from build123d import *

# Parameters (mm, degrees)
SKETCH1_W           = 81
SKETCH1_H           = 75
SKETCH1_R           = 1.585
BOSS_EXTRUDE1_DEPTH = 6.35


with BuildPart() as part:
    # Sketch1 → Boss-Extrude1 (new body)
    with BuildSketch(Plane(origin=(0, 0, 0), x_dir=(1, 0, 0), z_dir=(0, 1, 0))):
        with Locations((40.5, 37.5)):
            Rectangle(SKETCH1_W, SKETCH1_H)
        with Locations(Location((13.5, 5, 0), (0, 0, 270))):  # turned: the seam where the file's is
            Circle(SKETCH1_R, mode=Mode.SUBTRACT)
        with BuildLine():
            Line((6.175, 40), (74.825, 40))
            ThreePointArc((74.825, 40), (77.07006403, 40.92993597), (78, 43.175))
            Line((78, 43.175), (78, 66.825))
            ThreePointArc((78, 66.825), (77.07006403, 69.07006403), (74.825, 70))
            Line((74.825, 70), (6.175, 70))
            ThreePointArc((6.175, 70), (3.92993597, 69.07006403), (3, 66.825))
            Line((3, 66.825), (3, 43.175))
            ThreePointArc((3, 43.175), (3.92993597, 40.92993597), (6.175, 40))
        make_face(mode=Mode.SUBTRACT)
        with BuildLine():
            Line((61.83, 6.585), (65.17, 6.585))
            ThreePointArc((65.17, 6.585), (66.755, 5), (65.17, 3.415))
            Line((65.17, 3.415), (61.83, 3.415))
            ThreePointArc((61.83, 3.415), (60.245, 5), (61.83, 6.585))
        make_face(mode=Mode.SUBTRACT)
    extrude(amount=BOSS_EXTRUDE1_DEPTH)


solid = part.part
The listing builds one solid part. Answer for the finished solid, in the listing's coordinates (mm). A direction names the side the tool comes from. Coordinates: 2 decimals unless noted, no trailing zeros. Write each loop counter-clockwise with the first axis right and the second up, starting at its lowest first coordinate (ties: lowest second). Pieces come first, ordered by that corner, then holes. Notation, with made-up numbers: (3, 87.25) - (8, 87.25) arc R36 ccw to (8, 125.25) - close; hole circle Ø2 at (88, 59.5). An arc over 180 degrees is marked (long way). Put each result on its own line as item: value.
1. A flat-ended cylindrical pin translates along its axis: pin 1 Ø1.9 at (x, z) = (13.5, -5) entering from +Y. Find the tip coordinate at first contact, or state that the pin passes through.
Answer sheet:
pin 1: passes through
2. A tool of negligible diameter and unlimited length cuts with its end or side. For faces 5 (the face through (40, 6.35, -30)), 6 (the face through (63, 3, -6.585)), from which of +Z, -Z, +X, -X, +Y, -Y can it reach the whole face along a straight path? Write none if from no direction.
Answer sheet:
face 5: +Z, -Z, +X, -X, +Y
face 6: +Y, -Y
3. The part is cut by section B-B on x = 13.5. Give the vertices of the cut face in (y, z) (3 decimals).
Answer sheet:
outline: (0, -75) - (6.35, -75) - (6.35, -70) - (0, -70) - close; (0, -40) - (6.35, -40) - (6.35, -6.585) - (0, -6.585) - close; (0, -3.415) - (6.35, -3.415) - (6.35, 0) - (0, 0) - close
4. Determine the mould class of faces 1 (the face through (81, 3, -37)), 2 (the face through (40, 3, 0)), 3 (the face through (64, 3, -3.415)), 4 (the face through (3.95, 3.13, -69.09)) for opening direction X: pulls with the +X half, pulls with the -X half, needs draft (parallel to the pull), parting line crosses it, or undercut.
Answer sheet:
face 1: pulls with the +X half
face 2: needs draft
face 3: undercut
face 4: undercut
5. The part is cut by section A-A on z = -5. Give the vertices of the cut face in (x, y) (3 decimals).
Answer sheet:
outline: (0, 0) - (11.915, 0) - (11.915, 6.35) - (0, 6.35) - close; (15.085, 0) - (60.245, 0) - (60.245, 6.35) - (15.085, 6.35) - close; (66.755, 0) - (81, 0) - (81, 6.35) - (66.755, 6.35) - close
6. The part is cut by section D-D on y = 3.25. Give the vertices of the cut face in (x, z) (3 decimals).
Answer sheet:
outline: (0, -75) - (81, -75) - (81, 0) - (0, 0) - close; hole (3, -66.825) arc R3.175 ccw to (6.175, -70) - (74.825, -70) arc R3.175 ccw to (78, -66.825) - (78, -43.175) arc R3.175 ccw to (74.825, -40) - (6.175, -40) arc R3.175 ccw to (3, -43.175) - close; hole circle Ø3.17 at (13.5, -5); hole (61.83, -6.585) - (65.17, -6.585) arc R1.585 ccw to (65.17, -3.415) - (61.83, -3.415) arc R1.585 ccw to start
7. Find the intervals of material crossed by line 1 along X through (y, z) = (4, -5) (3 decimals); line 2 along Z through (x, y) = (62, 0.5) (3 decimals); line 3 along Z through (x, y) = (42.5, 2.75), in increasing order. Write a range as from..to.
Answer sheet:
line 1: x = 0..11.915, 15.085..60.245, 66.755..81
line 2: z = -75..-70, -40..-6.585, -3.415..0
line 3: z = -75..-70, -40..0
8. The part is cut by section C-C on x = 70. Give the vertices of the cut face in (y, z), plus the area to 3 significant figures.
Answer sheet:
outline: (0, -75) - (6.35, -75) - (6.35, -70) - (0, -70) - close; (0, -40) - (6.35, -40) - (6.35, 0) - (0, 0) - close
area: 286 mm^2
